Source: CAD feature listing. Evaluate the final solid. Frame: model axes, mm. A direction names the side the tool comes from. Coordinates: 2 decimals unless noted, no trailing zeros. Loops run counter-clockwise (first coordinate to the right, second up) from the corner with the lowest first, then second, coordinate; pieces in that order, holes last. Notation, with made-up numbers: M 23,64.5 L 78,64.5 A8 ccw 78,76.5 Z; hole C 67.25,82.5 d5. An arc over 180 degrees is marked long. Write each question's results on one line, items separated by ' | '. Start each with the question number.
from build123d import *

# Parameters (mm, degrees)
SKETCH_2_R          = 60
EXTRUDE_1_DEPTH     = 6
SKETCH_3_W          = 60
SKETCH_3_H          = 6.2
SKETCH_3_W_2        = 6.2
SKETCH_3_H_2        = 60
CUT_EXTRUDE_1_DEPTH = 6
FILLET_1_R          = 2


with BuildPart() as part:
    # 草图2 → 凸台-拉伸1 (new body)
    with BuildSketch(Plane(origin=(0, 0, 0), x_dir=(1, 0, 0), z_dir=(0, 1, 0))):
        with Locations(Location((0, 0, 0), (0, 0, 270))):
            Circle(SKETCH_2_R)
    extrude(amount=EXTRUDE_1_DEPTH)

    # 草图3 → 切除-拉伸1 (cut)
    with BuildSketch(Plane(origin=(0, 6, 0), x_dir=(1, 0, 0), z_dir=(0, 1, 0))):
        with Locations((68, 0)):
            Rectangle(SKETCH_3_W, SKETCH_3_H)
        Polygon((24.678026663, -29.062088707), (67.104433535, -71.488495578), (71.488495578, -67.104433535), (29.062088707, -24.678026663), align=None)
        with Locations((0, -68)):
            Rectangle(SKETCH_3_W_2, SKETCH_3_H_2)
        Polygon((-29.062088707, -24.678026663), (-71.488495578, -67.104433535), (-67.104433535, -71.488495578), (-24.678026663, -29.062088707), align=None)
        with Locations((-68, 0)):
            Rectangle(SKETCH_3_W, SKETCH_3_H)
        Polygon((-24.678026663, 29.062088707), (-67.104433535, 71.488495578), (-71.488495578, 67.104433535), (-29.062088707, 24.678026663), align=None)
        with Locations((0, 68)):
            Rectangle(SKETCH_3_W_2, SKETCH_3_H_2)
        Polygon((29.062088707, 24.678026663), (71.488495578, 67.104433535), (67.104433535, 71.488495578), (24.678026663, 29.062088707), align=None)
    extrude(amount=-CUT_EXTRUDE_1_DEPTH, mode=Mode.SUBTRACT)

    # 圆角1
    fillet_1_edges = [part.edges().sort_by_distance(p)[0] for p in [
        (29.062088707, 3, 24.678026663),
        (24.678026663, 3, 29.062088707),
        (38, 3, -3.1),
        (38, 3, 3.1),
        (24.678026663, 3, -29.062088707),
        (29.062088707, 3, -24.678026663),
        (-3.1, 3, -38),
        (3.1, 3, -38),
        (-29.062088707, 3, -24.678026663),
        (-24.678026663, 3, -29.062088707),
        (-38, 3, 3.1),
        (-38, 3, -3.1),
        (-24.678026663, 3, 29.062088707),
        (-29.062088707, 3, 24.678026663),
        (3.1, 3, 38),
        (-3.1, 3, 38),
    ]]
    fillet(fillet_1_edges, radius=FILLET_1_R)


solid = part.part
Item 1: Mould query, pull axis X, two halves, no side actions, for faces 4 (the flat face through (-37.42, 3.042, 33.036)), 5 (the cylindrical face through (-22.7, 2.96, -55.54)), 6 (the flat face through (50, 3, 3.1)). Classes: +X half, -X half, draft (parallel to the pull), parting line (faces both ways), or undercut.
Item 2: Access query for faces 1 (the flat face through (-3.1, 3, 50)), 2 (the flat face through (-3.1, 3, -50)), 3 (the flat face through (-33.036, 3.042, -37.42)). Directions: +Z, -Z, +X, -X, +Y, -Y. A direction counts if a zero-diameter tool reaches every point of the face in a straight line with its end or side. Return the directions, or none.
Item 3: First-contact query: pin 1 Ø1.5 at (x, y) = (19, 5) entering from -Z; pin 2 Ø1.5 at (y, z) = (4, 1) entering from +X; pin 3 Ø3 at (y, z) = (4, -54) entering from -X; pin 4 Ø1.5 at (x, z) = (32, 27) entering from -Y. Flat tips, straight axial feed; report the tip coordinate or a pass-through.
Item 4: Cut plane A-A (x = 32). Output: boundary loops of the cut face in (y, z).
Item 5: Cut plane C-C (z = -33). Output: boundary loops of the cut face in (x, y).
Item 6: Cut plane B-B (z = -50.5). Output: boundary loops of the cut face in (x, y).
Item 7: Cut plane D-D (x = -23). Output: boundary loops of the cut face in (y, z).
Item 8: Line query: probe 1 along Z at (x, y) = (36.5, 4.75); probe 2 along X at (y, z) = (4.75, -30); probe 3 along Z at (x, y) = (37.5, 1.5). Output: solid intervals per line, ascending.
Response values:
1) face 4: undercut | face 5: -X half | face 6: draft
2) face 1: +Z, +Y, -Y | face 2: -Z, +Y, -Y | face 3: +Y, -Y
3) pin 1: stops at z = -57.16 | pin 2: stops at x = 38.11 | pin 3: stops at x = -29.05 | pin 4: stops at y = 0
4) outline: M 0,-50.75 L 6,-50.75 L 6,-36.38 L 0,-36.38 Z; M 0,-27.62 L 6,-27.62 L 6,27.62 L 0,27.62 Z; M 0,36.38 L 6,36.38 L 6,50.75 L 0,50.75 Z
5) outline: M -50.11,0 L -37.38,0 L -37.38,6 L -50.11,6 Z; M -28.62,0 L 28.62,0 L 28.62,6 L -28.62,6 Z; M 37.38,0 L 50.11,0 L 50.11,6 L 37.38,6 Z
6) outline: M -32.4,0 L -3.1,0 L -3.1,6 L -32.4,6 Z; M 3.1,0 L 32.4,0 L 32.4,6 L 3.1,6 Z
7) outline: M 0,-55.42 L 6,-55.42 L 6,55.42 L 0,55.42 Z
8) probe 1: z = -47.62 to -40.88, -32.12 to 32.12, 40.88 to 47.62 | probe 2: x = -51.96 to -34.38, -25.74 to 25.74, 34.38 to 51.96 | probe 3: z = -46.84 to -41.88, -33.12 to 33.12, 41.88 to 46.84
